Source: CAD feature listing. Evaluate the final solid. Frame: model axes, mm. Coordinates: 2 decimals unless noted, no trailing zeros. Write each loop counter-clockwise with the first axis right and the second up, starting at its lowest first coordinate (ties: lowest second). Pieces come first, ordered by that corner, then holes. Notation, with made-up numbers: (-37, 47) - (7, 47) arc R9 cw to (7, 51) - close; hole circle Ø1 at (59, 3). An arc over 180 degrees is marked (long way). One line per question, with ' | ' between items. Start each with the question number.
Q1. Cut plane A-A, the plane z = -74. Return loops of the section in (x, y), plus the area to 3 significant figures.
Q2. Cut plane B-B, the plane z = 27.5. Return loops of the section in (x, y), plus the area to 3 significant figures.
Q3. Line query: line 1 (X direction, y = 2, z = 125); line 2 (Y direction, x = -26.5, z = -10); line 3 (Y direction, x = -12, z = -167). Output: solid intervals per line, ascending.
Q4. Contact query for flat-ended pins moving along their axis: P1, Ø12, axis at y = -8.5, z = 109.5, coming from the -X side; P2, Ø2, axis at x = -6, z = 82, coming from the +Y side; P3, Ø1.5, axis at y = 19.5, z = -40, coming from the -X side. Output: stop coordinate, or through.
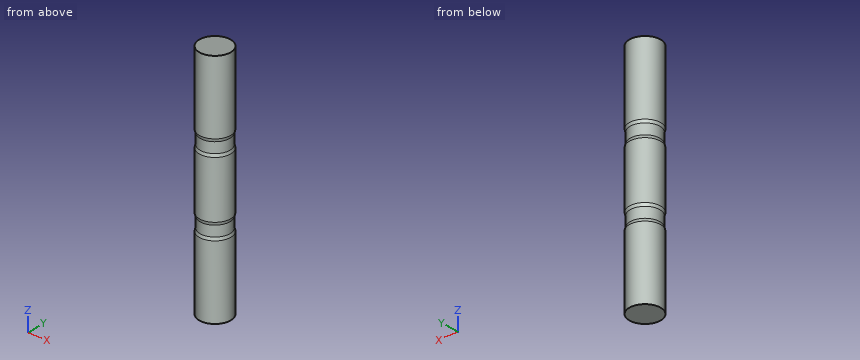
```python
from build123d import *

# Parameters (mm, degrees)
SKETCH1_R           = 30
BOSS_EXTRUDE1_DEPTH = 225


with BuildPart() as part:
    # Sketch1 → Boss-Extrude1 (new body, symmetric)
    with BuildSketch(Plane.XY):
        Circle(SKETCH1_R)
    extrude(amount=BOSS_EXTRUDE1_DEPTH, both=True)

    # Sketch3 → Cut-Revolve1 (revolve, cut)
    with BuildSketch(Plane(origin=(0, 0, 0), x_dir=(0, 0, -1), z_dir=(1, 0, 0))):
        Polygon((-85.598076211, 30), (-80, 28.5), (-60, 28.5), (-54.401923789, 30), align=None)
        Polygon((85.598076211, 30), (54.401923789, 30), (60, 28.5), (80, 28.5), align=None)
    revolve(axis=Axis((0, 0, 225), (0, 0, -1)), mode=Mode.SUBTRACT)


solid = part.part
```
Reply:
1) outline: circle Ø57 at (0, 0) | area: 2,550 mm^2
2) outline: circle Ø60 at (0, 0) | area: 2,830 mm^2
3) line 1: x = -29.93 to 29.93 | line 2: y = -14.06 to 14.06 | line 3: y = -27.5 to 27.5
4) P1: stops at x = -29.9 | P2: stops at y = 28.75 | P3: stops at x = -23.42
